from build123d import *

# Parameters (mm, degrees)
CUT_EXTRUDE1_DEPTH      = 20.195683783
CUT_EXTRUDE1_DEPTH_BACK = 20.195683783
SKETCH2_R               = 1.5


with BuildPart() as part:
    # Sketch1 → Revolve1 (revolve)
    with BuildSketch(Plane.XY, mode=Mode.PRIVATE) as revolve1_sk:
        Polygon((0, 0), (-6.25, 0), (-6.25, -1), (-7, -1), (-7, -16.446102149), (-6.2, -16.446102149), (-4.25, -11.088521181), (-4.25, -5.446102149), (0, -2.892444518), align=None)
    revolve(revolve1_sk.sketch.rotate(Axis((0, 0, 0), (0, -1, 0)), 270), axis=Axis((0, 0, 0), (0, -1, 0)))

    # Sketch2 → Cut-Extrude1 (cut, two sides: drawn at the far end of the back side and taken through both)
    with BuildSketch(Plane(origin=(0, 0, 0), x_dir=(0, 0, -1), z_dir=(1, 0, 0)).offset(-CUT_EXTRUDE1_DEPTH_BACK)):
        with Locations((0, -9.446102149)):
            Circle(SKETCH2_R)
    extrude(amount=CUT_EXTRUDE1_DEPTH + CUT_EXTRUDE1_DEPTH_BACK, mode=Mode.SUBTRACT)


solid = part.part
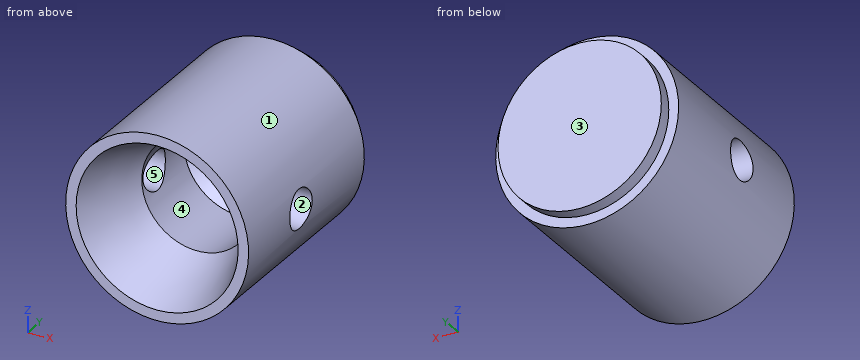
Geometry: final body of the model. Coordinates: model frame, mm. Face numbers are marked on the shaded views. A direction names the side the tool comes from. Round coordinates to 2 decimals unless told otherwise and drop trailing zeros. Write each loop counter-clockwise with the first axis right and the second up, starting at its lowest first coordinate (ties: lowest second). Pieces come first, ordered by that corner, then holes. Notation, with made-up numbers: M 49,2.25 L 56,2.25 A29 ccw 56,41.25 Z; hole C -22,34 d10. An arc over 180 degrees is marked long. Write item = value, one per line.
Item 1: Pin query (flat end, axial travel): P1, Ø1.8, axis at y = -9.45, z = 0, coming from the +X side; P2, Ø6, axis at x = -4.5, y = -3, coming from the -Z side; P3, Ø6, axis at x = -4, z = -2.5, coming from the -Y side. Return the tip coordinate at first contact, or that it passes through.
Findings:
P1 = through
P2 = -6.84
P3 = -16.45
Item 2: Section query A-A on y = -6. Return loops of the section in (x, z).
Findings:
outline = C 0,0 d14; hole C 0,0 d8.5
Item 3: Access query for the marked faces 4 and 5. Directions: +Z, -Z, +X, -X, +Y, -Y. A direction counts if a zero-diameter tool reaches every point of the face in a straight line with its end or side. Return the directions, or none.
Findings:
face_4 = -Y
face_5 = +X, -X
Item 4: Material intervals for line 1 along Y through (x, z) = (6.75, 0); line 2 along Y through (x, z) = (1.5, 1); line 3 along Z through (x, y) = (-3, -12.5), sorted ascending. Write a range as [from, to].
Findings:
line_1 = [-16.45, -10.95], [-7.95, -1]
line_2 = [-3.98, 0]
line_3 = [-6.32, -3.7], [3.7, 6.32]
Item 5: Pull-direction query (Z, two-part tool) for the marked faces 1, 2 and 3; classes: pulls with the +Z half, pulls with the -Z half, needs draft (parallel to the pull), parting line crosses it, or undercut.
Findings:
face_1 = parting line crosses it
face_2 = undercut
face_3 = needs draft
Item 6: Section query B-B on y = -9. Return loops of the section in (x, z), then the cut area to 3 significant figures.
Findings:
outline = M -6.85,-1.43 A7 ccw 6.85,-1.43 L 4,-1.43 A4.25 cw -4,-1.43 Z; M -6.85,1.43 L -4,1.43 A4.25 cw 4,1.43 L 6.85,1.43 A7 ccw Z
area = 81.3 mm^2
Item 7: Section query C-C on z = 0.75. State how many separate pieces and enclosed holes the cut face has, then the cut area to 3 significant figures.
Findings:
separate_pieces = 3
enclosed_holes = 0
area = 101 mm^2
